```python
from build123d import *

# Parameters (mm, degrees)
F0_W     = 76.2
F0_H     = 76.2
F0_W_2   = 63.5
F0_H_2   = 63.5
F1_DEPTH = 609.6
F2_W     = 76.2
F2_H     = 152.4
F3_DEPTH = 12.7
F4_R     = 4.7625
F5_DEPTH = 25.4


with BuildPart() as f1:
    # F0 (on Top) → F1 (new body)
    with BuildSketch(Plane.XY):
        with Locations((38.1, 38.1)):
            Rectangle(F0_W, F0_H)
        with Locations((38.1, 38.1)):
            Rectangle(F0_W_2, F0_H_2, mode=Mode.SUBTRACT)
    extrude(amount=F1_DEPTH)

    # F2 (on face) → F3 (join)
    with BuildSketch(Plane.XY.offset(609.6)):
        with Locations((38.1, 38.1)):
            Rectangle(F2_W, F2_H)
    extrude(amount=F3_DEPTH)

    # F4 (on face) → F5 (cut)
    with BuildSketch(Plane.XY.offset(622.3)):
        with Locations((50.8, 25.4)):
            Circle(F4_R)
        with Locations((25.4, 25.4)):
            Circle(F4_R)
    extrude(amount=-F5_DEPTH, mode=Mode.SUBTRACT)


solid = f1.part
```
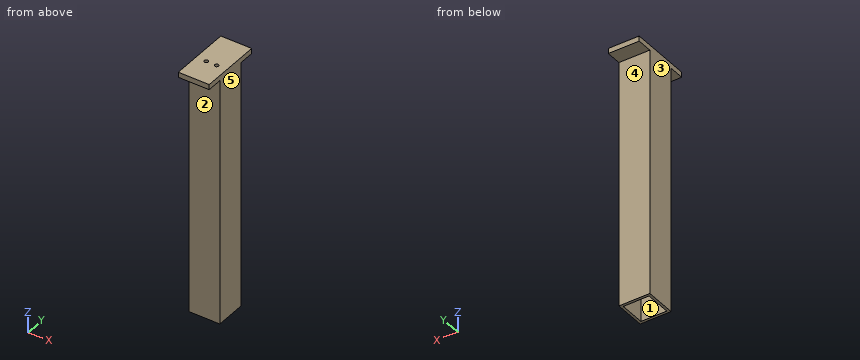
Can you work these out from the model? Positions are in its coordinate system, mm. Face numbers are marked on the shaded views. A direction names the side the tool comes from. Round coordinates to 2 decimals unless told otherwise and drop trailing zeros. Loops run counter-clockwise (first coordinate to the right, second up) from the corner with the lowest first, then second, coordinate; pieces in that order, holes last. Notation, with made-up numbers: M -2.5,58.25 L 17.5,58.25 A20 cw 17.5,77.25 Z; hole C -37.75,-39.75 d3. An arc over 180 degrees is marked long. Answer as a JSON object with one key per item and string values. Group by question number.
Q1. Will these pins go through, and if not, where does the flat tip stop? pin 1 (3 mm diameter, centred on x = 12, y = 60, fed in from -Z); pin 2 (7.5 mm diameter, centred on x = 50.8, y = 25.4, fed in from -Z); pin 3 (3 mm diameter, centred on x = 60.5, z = 462, fed in from -Y); pin 4 (6 mm diameter, centred on x = 27.5, y = 24.5, fed in from +Z).
Q2. Please list where these lines run through material, in increasing order: L1, parallel to Y at x = 40, z = 255; L2, parallel to Y at x = 50, z = 615; L3, parallel to X at y = 25, z = 617.
Q3. Imagine slicing it at C-C, the plane y = 56. Please give me the cut outline in (x, z).
Q4. Imagine slicing it at D-D, the plane y = -25. Please give me the cut outline in (x, z), then the cut area to 3 significant figures.
Q5. On a 3-axis mill with a long thin cutter (end or side, diameter ignored), from which of +Z, -Z, +X, -X, +Y, -Y can I reach the whole of each face in a straight line? I mean the marked faces 4 and 5. Say none if no direction works.
Q6. We'd pull the mould along Y, two halves only. Please class the marked faces 1, 2 and 3: +Y half, -Y half, draft (parallel to the pull), parting line (faces both ways), or undercut.
Q7. Imagine slicing it at A-A, the plane z = 73. Please give me the cut outline in (x, y).
Q8. Imagine slicing it at B-B, the plane x = 63. Please give me the cut outline in (y, z), then the cut area to 3 significant figures.
Findings:
{
 "1": {"pin 1": "stops at z = 609.6", "pin 2": "passes through", "pin 3": "stops at y = 0", "pin 4": "stops at z = 622.3"},
 "2": {"L1": "y = 0 to 6.35, 69.85 to 76.2", "L2": "y = -38.1 to 20.71, 30.09 to 114.3", "L3": "x = 0 to 20.65, 30.15 to 46.05, 55.55 to 76.2"},
 "3": {"outline": "M 0,0 L 6.35,0 L 6.35,609.6 L 69.85,609.6 L 69.85,0 L 76.2,0 L 76.2,622.3 L 0,622.3 Z"},
 "4": {"outline": "M 0,609.6 L 76.2,609.6 L 76.2,622.3 L 0,622.3 Z", "area": "968 mm2"},
 "5": {"face 4": "-Z, +X, -X, +Y", "face 5": "+Z, -Z, +X, +Y, -Y"},
 "6": {"face 1": "undercut", "face 2": "-Y half", "face 3": "draft"},
 "7": {"outline": "M 0,0 L 76.2,0 L 76.2,76.2 L 0,76.2 Z; hole M 6.35,6.35 L 69.85,6.35 L 69.85,69.85 L 6.35,69.85 Z"},
 "8": {"outline": "M -38.1,609.6 L 0,609.6 L 0,0 L 6.35,0 L 6.35,609.6 L 69.85,609.6 L 69.85,0 L 76.2,0 L 76.2,609.6 L 114.3,609.6 L 114.3,622.3 L -38.1,622.3 Z", "area": "9,680 mm2"}
}
